Read the model definition and answer for the solid it produces. Units are mm, in the model's axes. A direction names the side the tool comes from. Coordinates: 2 decimals unless noted, no trailing zeros. Order: outer loops, then holes, each group sorted by start corner. A loop starts at its lowest first (then second) coordinate and runs counter-clockwise, first axis right, second up. Notation, with made-up numbers: (29.25, 25) - (34.25, 25) arc R23 ccw to (34.25, 55) - close; hole circle Ø1 at (27.25, 79). An arc over 180 degrees is marked (long way). Use one line per item in the form item = value. Start each with the question number.
from build123d import *

# Parameters (mm, degrees)
ESQUISSE1_W             = 45
ESQUISSE1_H             = 35
BOSS_EXTRU_1_DEPTH      = 8.1
ESQUISSE2_W             = 24
ESQUISSE2_H             = 10.2
BOSS_EXTRU_2_DEPTH      = 8.1
ESQUISSE3_R             = 1
ENL_V_MAT_EXTRU_1_DEPTH = 58.581333781
CHANFREIN1_SIZE         = 4
CONG_1_R                = 2.5


with BuildPart() as part:
    # Esquisse1 → Boss.-Extru.1 (new body)
    with BuildSketch(Plane.XY):
        with Locations((22.5, 17.5)):
            Rectangle(ESQUISSE1_W, ESQUISSE1_H)
    extrude(amount=BOSS_EXTRU_1_DEPTH)

    # Esquisse2 → Boss.-Extru.2 (add)
    with BuildSketch(Plane.XY.offset(8.1)):
        with Locations((-12, 29.9)):
            Rectangle(ESQUISSE2_W, ESQUISSE2_H)
    extrude(amount=-BOSS_EXTRU_2_DEPTH)

    # Esquisse3 → Enlèv. mat.-Extru.1 (cut, through all)
    with BuildSketch(Plane.XY.offset(8.1)):
        with Locations((-4, 27.2)):
            Circle(ESQUISSE3_R)
        with Locations((-21, 27.2)):
            Circle(ESQUISSE3_R)
        with Locations((2.5, 20.9)):
            Circle(ESQUISSE3_R)
        with Locations((2.5, 3.9)):
            Circle(ESQUISSE3_R)
    extrude(amount=-ENL_V_MAT_EXTRU_1_DEPTH, mode=Mode.SUBTRACT)

    # Chanfrein1
    chanfrein1_edges = [part.edges().sort_by_distance(p)[0] for p in [
        (0, 24.8, 4.05),
    ]]
    chamfer(chanfrein1_edges, length=CHANFREIN1_SIZE)

    # Congé1
    cong_1_edges = [part.edges().sort_by_distance(p)[0] for p in [
        (-24, 24.8, 4.05),
        (-24, 35, 4.05),
        (0, 0, 4.05),
    ]]
    fillet(cong_1_edges, radius=CONG_1_R)


solid = part.part
Q1. Which of the six approach directions +Z, -Z, +X, -X, +Y, -Y give full straight-line access (tool end or side, diameter ignored) to faces 1 (the flat face through (0, 12, 4)), 2 (the cylindrical face through (1.7, 3.3, 4.1))?
Q2. For a pull along Y with two mould halves and no side action, classify faces 3 (the cylindrical face through (2.37, 21.89, 4.11)), 4 (the cylindrical face through (-23.287, 34.248, 3.993)), 5 (the flat face through (-13, 24.8, 4)) as +Y half, -Y half, draft (parallel to the pull), parting line (faces both ways), or undercut.
Q3. A cutting plane is placed at B-B (y = 8.5). Give the vertices of the cut face in (x, z).
Q4. Given P1, Ø1.2, axis at x = -21, y = 27.2, coming from the +Z side; P2, Ø2.5, axis at y = 7, z = 3, coming from the -X side; P3, Ø4, axis at y = 22.5, z = 6, coming from the -X side, each flat-ended and moving along its own axis, determine where each tip first touches the part or whether it passes through.
Q5. Consider probe 1 along Y at (x, z) = (2.5, 2.5); probe 2 along Y at (x, z) = (-4, 3); probe 3 along X at (y, z) = (17, 5.25). Determine where each line is inside the solid, lowest interval first.
Q6. A cutting plane is placed at A-A (z = 2.5). Give the vertices of the cut face in (x, y).
Q7. A cutting plane is placed at C-C (x = -13.5). Give the vertices of the cut face in (y, z).
Result sheet:
q1.face_1 = +Z, -Z, -X, -Y
q1.face_2 = +Z, -Z
q2.face_3 = undercut
q2.face_4 = +Y half
q2.face_5 = -Y half
q3.outline = (0, 0) - (45, 0) - (45, 8.1) - (0, 8.1) - close
q4.P1 = through
q4.P2 = 0
q4.P3 = -3.7
q5.probe_1 = 0 to 2.9, 4.9 to 19.9, 21.9 to 35
q5.probe_2 = 24.8 to 26.2, 28.2 to 35
q5.probe_3 = 0 to 45
q6.outline = (-24, 27.3) arc R2.5 ccw to (-21.5, 24.8) - (-4, 24.8) - (0, 20.8) - (0, 2.5) arc R2.5 ccw to (2.5, 0) - (45, 0) - (45, 35) - (-21.5, 35) arc R2.5 ccw to (-24, 32.5) - close; hole circle Ø2 at (-21, 27.2); hole circle Ø2 at (-4, 27.2); hole circle Ø2 at (2.5, 3.9); hole circle Ø2 at (2.5, 20.9)
q7.outline = (24.8, 0) - (35, 0) - (35, 8.1) - (24.8, 8.1) - close
